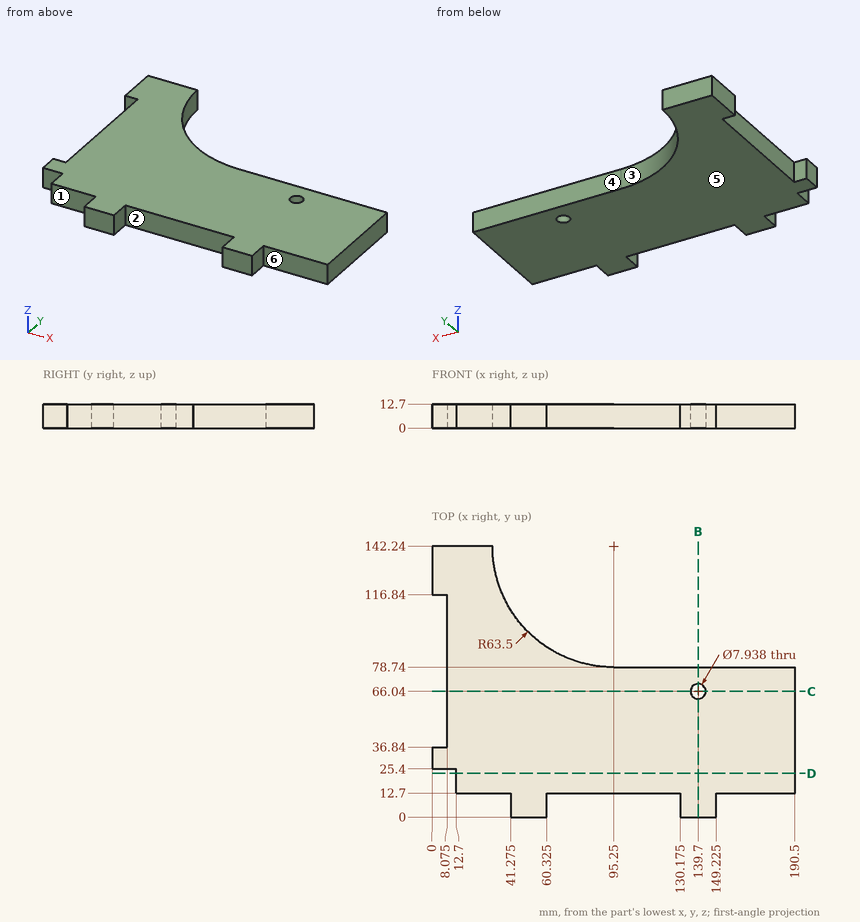
Study the drawing (mm; zero at the part's minimum x, y, z) and answer. A direction names the side the tool comes from. Give positions to 0.01 mm unless a question says otherwise; leave off trailing zeros. Loops run counter-clockwise (first coordinate to the right, second up) from the corner with the lowest first, then second, coordinate; pieces in that order, holes last. Notation, with made-up numbers: M -27.75,83.5 L 18.25,83.5 A31 cw 18.25,114.5 Z; hole C 60.5,-16.75 d7. An arc over 180 degrees is marked long. Answer as CSV lines item,"result".
Item 1: The part is cut by section B-B (x = 139.7). Give the vertices of the cut face in (y, z).
Values follow:
outline,"M 0,0 L 62.07,0 L 62.07,12.7 L 0,12.7 Z; M 70.01,0 L 78.74,0 L 78.74,12.7 L 70.01,12.7 Z"
Item 2: Straight lines are drawn through the part: line 1 along Y through (x, z) = (139.7, 4); line 2 along Y through (x, z) = (127, 4.5); line 3 along Y through (x, z) = (93, 10.25). For each, find the intervals that lie inside material, in ascending order. Write a range as [from, to].
Values follow:
line 1,"y = [0, 62.07], [70.01, 78.74]"
line 2,"y = [12.7, 78.74]"
line 3,"y = [12.7, 78.78]"
Item 3: Given pin 1 Ø7 at (x, y) = (139.7, 66.04) entering from +Z; pin 2 Ø4 at (x, z) = (143, 8) entering from +Y; pin 3 Ø4 at (y, z) = (3.5, 7) entering from -X (1 decimal); pin 4 Ø1 at (x, z) = (112, 5) entering from -Y, each flat-ended and moving along its own axis, determine where each tip first touches the part or whether it passes through.
Values follow:
pin 1,"passes through"
pin 2,"stops at y = 78.74"
pin 3,"stops at x = 41.3"
pin 4,"stops at y = 12.7"
Item 4: The part is cut by section C-C (y = 66.04). Give the vertices of the cut face in (x, z) (1 decimal), and give its area (3 significant figures).
Values follow:
outline,"M 8.1,0 L 135.7,0 L 135.7,12.7 L 8.1,12.7 Z; M 143.7,0 L 190.5,0 L 190.5,12.7 L 143.7,12.7 Z"
area,"2,220 mm^2"
Item 5: Which of the six approach directions +Z, -Z, +X, -X, +Y, -Y give full straight-line access (tool end or side, diameter ignored) to the marked faces 4, 5 and 6?
Values follow:
face 4,"+Z, -Z, +X, +Y"
face 5,"-Z, +X, -X, +Y, -Y"
face 6,"+Z, -Z, +X, -Y"
Item 6: The mould has two halves that part along X. Classify the marked faces 1, 2 and 3: released by +X, released by -X, zero draft, split by the parting line, or undercut.
Values follow:
face 1,"zero draft"
face 2,"undercut"
face 3,"released by +X"
Item 7: The part is cut by section D-D (y = 23). Give the vertices of the cut face in (x, z).
Values follow:
outline,"M 12.7,0 L 190.5,0 L 190.5,12.7 L 12.7,12.7 Z"
